```python
from build123d import *

# Parameters (mm, degrees)
SKETCH1_W           = 252
SKETCH1_H           = 252
BOSS_EXTRUDE1_DEPTH = 4
SKETCH2_W           = 252
SKETCH2_H           = 29
SKETCH2_W_2         = 29
SKETCH2_H_2         = 252
BOSS_EXTRUDE2_DEPTH = 4
SKETCH3_W           = 260
SKETCH3_H           = 260
SKETCH3_W_2         = 252
SKETCH3_H_2         = 252
BOSS_EXTRUDE3_DEPTH = 24


with BuildPart() as part:
    # Sketch1 → Boss-Extrude1 (new body)
    with BuildSketch(Plane(origin=(0, 0, 0), x_dir=(1, 0, 0), z_dir=(0, 1, 0))):
        Rectangle(SKETCH1_W, SKETCH1_H)
    extrude(amount=BOSS_EXTRUDE1_DEPTH)

    # Sketch2 → Boss-Extrude2 (add)
    with BuildSketch(Plane(origin=(0, 4, 0), x_dir=(1, 0, 0), z_dir=(0, 1, 0))):
        Rectangle(SKETCH2_W, SKETCH2_H)
        Rectangle(SKETCH2_W_2, SKETCH2_H_2)
    extrude(amount=BOSS_EXTRUDE2_DEPTH)

    # Sketch3 → Boss-Extrude3 (add)
    with BuildSketch(Plane.XZ):
        Rectangle(SKETCH3_W, SKETCH3_H)
        Rectangle(SKETCH3_W_2, SKETCH3_H_2, mode=Mode.SUBTRACT)
    extrude(amount=-BOSS_EXTRUDE3_DEPTH)


solid = part.part
```
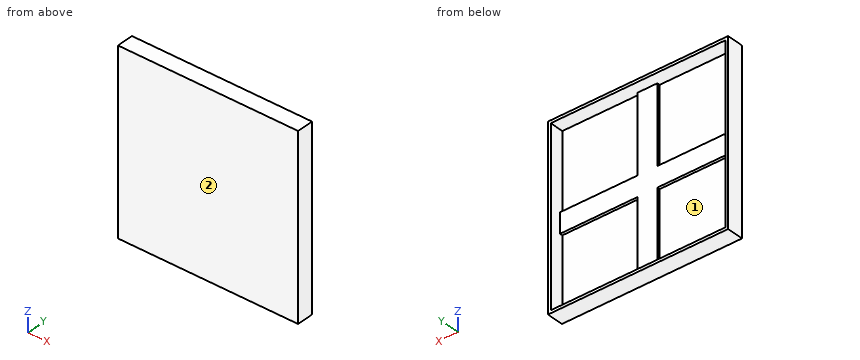
The model under review builds one solid part; all positions refer to its coordinate system, in mm. Face numbers are marked on the shaded views. Round coordinates to 2 decimals unless told otherwise and drop trailing zeros. Order: outer loops, then holes, each group sorted by start corner. A loop starts at its lowest first (then second) coordinate and runs counter-clockwise, first axis right, second up.
(1) Wall thickness on L1, parallel to X at y = 4.5, z = 95.5; L2, parallel to Z at x = 65.5, y = 11.5: over which ranges is each line inside the solid? List them lowest first.
Working result:
L1: x = -130 to -126, -14.5 to 14.5, 126 to 130
L2: z = -130 to -126, 126 to 130
(2) For P1, Ø6, axis at x = 94, z = 58.5, coming from the +Y side, flat-tipped, find the tip position at first contact; note if it passes through.
Working result:
P1: stops at y = 4
(3) Take a section at C-C, the plane x = 9. State the section outline as (y, z) points, plus the area to 3 significant figures.
Working result:
outline: (0, -130) - (24, -130) - (24, -126) - (8, -126) - (8, 126) - (24, 126) - (24, 130) - (0, 130) - close
area: 2,210 mm2
(4) Mouldability with a two-part tool opening along Z and no side actions: class the marked faces 1 and 2 as released by +Z, released by -Z, zero draft, split by the parting line, or undercut.
Working result:
face 1: undercut
face 2: zero draft
(5) Take a section at B-B, the plane z = 63.5. State the section outline as (x, y) points.
Working result:
outline: (-130, 0) - (130, 0) - (130, 24) - (126, 24) - (126, 4) - (14.5, 4) - (14.5, 8) - (-14.5, 8) - (-14.5, 4) - (-126, 4) - (-126, 24) - (-130, 24) - close
(6) Take a section at A-A, the plane y = 19. State the section outline as (x, z) points.
Working result:
outline: (-130, -130) - (130, -130) - (130, 130) - (-130, 130) - close; hole (-126, -126) - (126, -126) - (126, 126) - (-126, 126) - close
(7) Take a section at D-D, the plane x = 63. State the section outline as (y, z) points, plus the area to 3 significant figures.
Working result:
outline: (0, -130) - (24, -130) - (24, -126) - (4, -126) - (4, -14.5) - (8, -14.5) - (8, 14.5) - (4, 14.5) - (4, 126) - (24, 126) - (24, 130) - (0, 130) - close
area: 1,320 mm2
